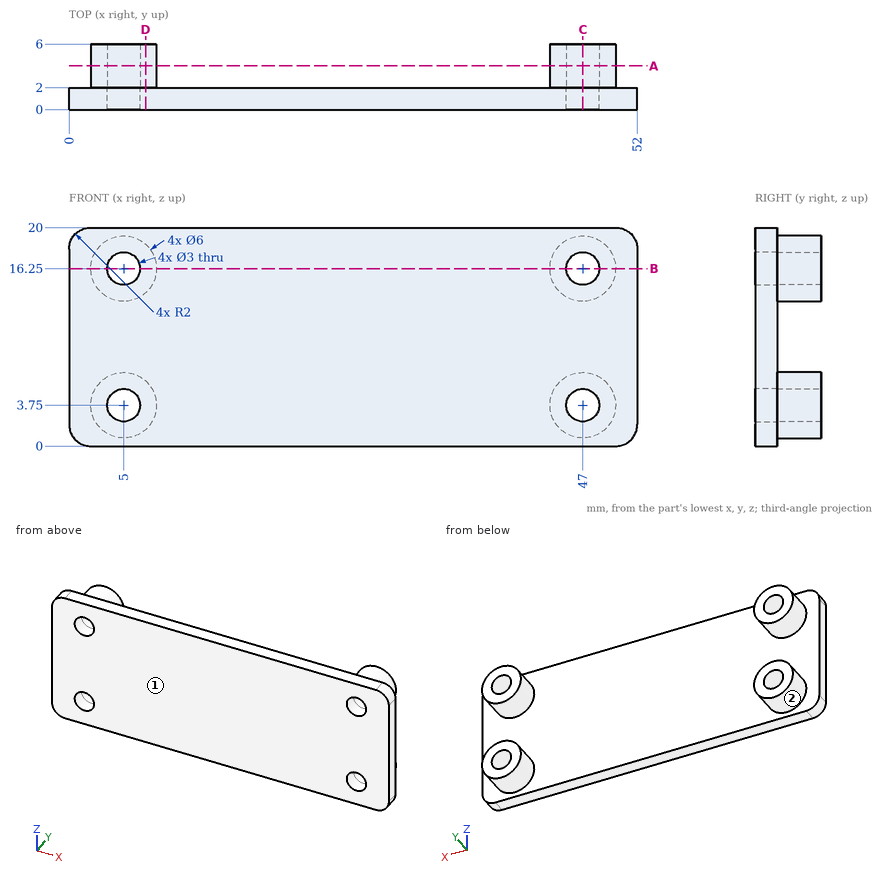
Source: three-view drawing plus pictorial views. Frame: mm from the lowest corner of the part. Give positions to 0.01 mm unless a question says otherwise; leave off trailing zeros. Order: outer loops, then holes, each group sorted by start corner. A loop starts at its lowest first (then second) coordinate and runs counter-clockwise, first axis right, second up. Notation, with made-up numbers: (81.5, 59.25) - (130.5, 59.25) arc R22 cw to (130.5, 82.25) - close; hole circle Ø4 at (20, 74.25). An arc over 180 degrees is marked (long way). Answer as a JSON object with one key per item and string values. Group by question number.
Q1. Cut plane C-C, the plane x = 47. Output: boundary loops of the cut face in (y, z).
Q2. First-contact query: pin 1 Ø6 at (x, z) = (26.5, 6.5) entering from +Y. Flat tip, straight axial feed; report the tip coordinate or a pass-through.
Q3. Line query: probe 1 along X at (y, z) = (5.15, 16.25); probe 2 along X at (y, z) = (1.45, 16.25); probe 3 along X at (y, z) = (2.3, 2.5). Output: solid intervals per line, ascending.
Q4. Mould query, pull axis Z, two halves, no side actions, for the marked faces 1 and 2. Classes: pulls with the +Z half, pulls with the -Z half, needs draft (parallel to the pull), parting line crosses it, or undercut.
Q5. Cut plane B-B, the plane z = 16.25. Output: boundary loops of the cut face in (x, y).
Q6. Cut plane A-A, the plane y = 4. Output: boundary loops of the cut face in (x, z).
Q7. Cut plane D-D, the plane x = 7. Output: boundary loops of the cut face in (y, z), then the cut area to 3 significant figures.
Results:
{
 "1": {"outline": "(0, 0) - (2, 0) - (2, 0.75) - (6, 0.75) - (6, 2.25) - (0, 2.25) - close; (0, 5.25) - (6, 5.25) - (6, 6.75) - (2, 6.75) - (2, 13.25) - (6, 13.25) - (6, 14.75) - (0, 14.75) - close; (0, 17.75) - (6, 17.75) - (6, 19.25) - (2, 19.25) - (2, 20) - (0, 20) - close"},
 "2": {"pin 1": "y = 2"},
 "3": {"probe 1": "2 to 3.5, 6.5 to 8, 44 to 45.5, 48.5 to 50", "probe 2": "0 to 3.5, 6.5 to 45.5, 48.5 to 52", "probe 3": "2.27 to 4.17, 5.83 to 7.73, 44.27 to 46.17, 47.83 to 49.73"},
 "4": {"face 1": "needs draft", "face 2": "undercut"},
 "5": {"outline": "(0, 0) - (3.5, 0) - (3.5, 6) - (2, 6) - (2, 2) - (0, 2) - close; (6.5, 0) - (45.5, 0) - (45.5, 6) - (44, 6) - (44, 2) - (8, 2) - (8, 6) - (6.5, 6) - close; (48.5, 0) - (52, 0) - (52, 2) - (50, 2) - (50, 6) - (48.5, 6) - close"},
 "6": {"outline": "circle Ø6 at (5, 3.75); circle Ø6 at (5, 16.25); circle Ø6 at (47, 3.75); circle Ø6 at (47, 16.25); hole circle Ø3 at (5, 3.75); hole circle Ø3 at (5, 16.25); hole circle Ø3 at (47, 3.75); hole circle Ø3 at (47, 16.25)"},
 "7": {"outline": "(0, 0) - (2, 0) - (2, 1.51) - (6, 1.51) - (6, 5.99) - (2, 5.99) - (2, 14.01) - (6, 14.01) - (6, 18.49) - (2, 18.49) - (2, 20) - (0, 20) - close", "area": "75.8 mm^2"}
}
